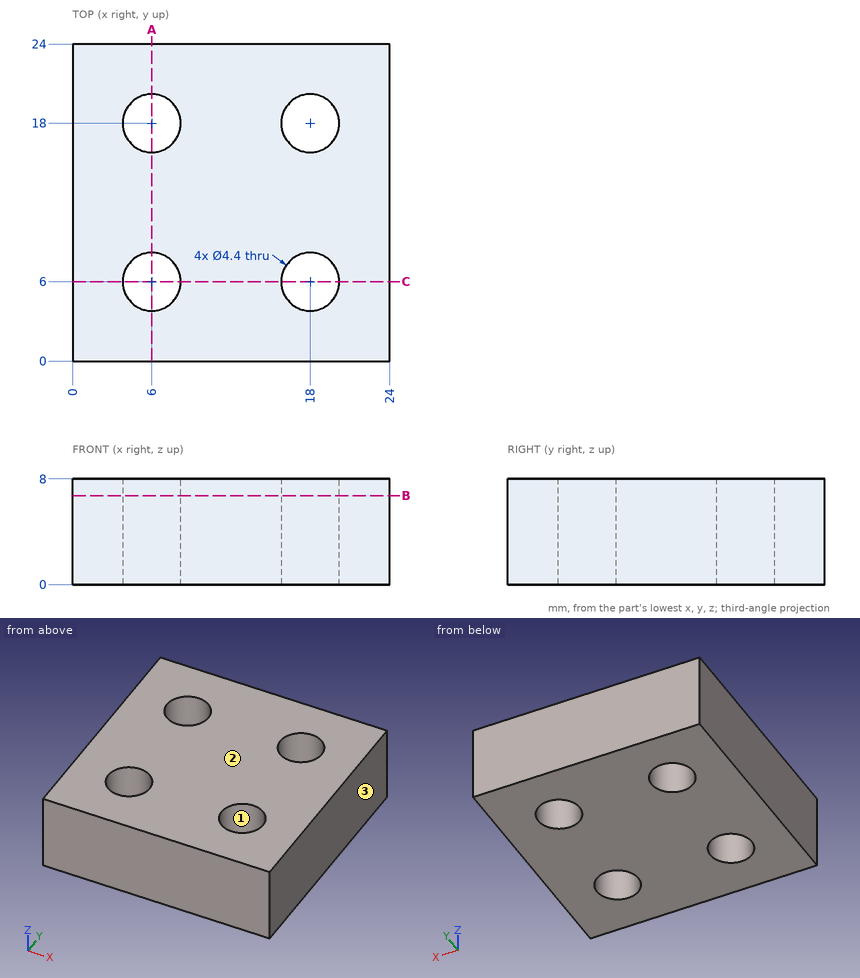
Job drawing, mm, ordinate dimensions from the low corner. One solid piece. Round coordinates to 2 decimals unless told otherwise and drop trailing zeros. Loops run counter-clockwise (first coordinate to the right, second up) from the corner with the lowest first, then second, coordinate; pieces in that order, holes last. Notation, with made-up numbers: (37, 1) -> (43, 1) arc R12 ccw to (43, 18) -> close; hole circle Ø10 at (72.25, 53). An arc over 180 degrees is marked (long way). Use CSV: the item, a comma, the result in double quotes. Start each with the question number.
Q1. Mould opens along X. For the marked faces 1, 2 and 3 say: +X half, -X half, draft (parallel to the pull), parting line (faces both ways), or undercut.
Q2. Drill centre lines: L1, parallel to Y at x = 6, z = 3; L2, parallel to X at y = 4, z = 1; L3, parallel to Y at x = 7.25, z = 5.5. Where is each one in solid material? Low to high.
Q3. Saw through at A-A on x = 6. Give the cut face in (y, z).
Q4. Saw through at B-B on z = 6.75. Give the cut face in (x, y).
Q5. Flat gauge pins, fed straight in: pin 1 Ø4 at (x, y) = (6, 6) entering from -Z; pin 2 Ø4 at (y, z) = (13.5, 4.5) entering from -X. Where does each tip first touch, or does it go through?
Solutions:
1,face 1,"undercut"
1,face 2,"draft"
1,face 3,"+X half"
2,L1,"y = 0 to 3.8, 8.2 to 15.8, 20.2 to 24"
2,L2,"x = 0 to 5.08, 6.92 to 17.08, 18.92 to 24"
2,L3,"y = 0 to 4.19, 7.81 to 16.19, 19.81 to 24"
3,outline,"(0, 0) -> (3.8, 0) -> (3.8, 8) -> (0, 8) -> close; (8.2, 0) -> (15.8, 0) -> (15.8, 8) -> (8.2, 8) -> close; (20.2, 0) -> (24, 0) -> (24, 8) -> (20.2, 8) -> close"
4,outline,"(0, 0) -> (24, 0) -> (24, 24) -> (0, 24) -> close; hole circle Ø4.4 at (6, 6); hole circle Ø4.4 at (6, 18); hole circle Ø4.4 at (18, 6); hole circle Ø4.4 at (18, 18)"
5,pin 1,"passes through"
5,pin 2,"stops at x = 0"
